Geometry check sheet. Reference: the model listing, model coordinates, mm. A direction names the side the tool comes from. Round coordinates to 2 decimals unless told otherwise and drop trailing zeros. Loops run counter-clockwise (first coordinate to the right, second up) from the corner with the lowest first, then second, coordinate; pieces in that order, holes last. Notation, with made-up numbers: (1, 77.25) - (35, 77.25) arc R16 cw to (35, 83.25) - close; hole circle Ø3 at (33, -10). An arc over 180 degrees is marked (long way). Write item = value, one per line.
Autodesk Inventor part; units mm, degrees
ref_plane "Work Plane1" through (0, 0, -15) normal (0, 0, 1) x (1, 0, 0)
ref_plane "YZ Plane" through (0, 0, 0) normal (1, 0, 0) x (0, 1, 0)
ref_plane "XZ Plane" through (0, 0, 0) normal (0, 1, 0) x (-1, 0, 0)
sketch "Sketch1" plane through (0, 0, 0) normal (0, 0, 1) x (1, 0, 0)
  line L0 (0, 0) -> (25, 0)
  line L1 (25, 0) -> (25, 40)
  line L2 (25, 40) -> (0, 40)
  line L3 (0, 40) -> (0, 0)
  dimension "d1" = 25
  dimension "d2" = 40
  dimension "d3" = 25
extrude "Extrusion1" add sketch "Sketch1" against normal blind 30
sketch "Sketch2" plane through (25, 0, 0) normal (1, 0, 0) x (0, 0, -1)
  line L0 (0, 0) -> (30, 0)
  circle A0 centre (15, 6.56) radius 2.46
extrude "Extrusion2" cut sketch "Sketch2" against normal blind 30
sketch "Sketch3" plane through (0, 0, 0) normal (-1, 0, 0) x (0, 0, 1)
  line L0 (0, 0) -> (-30, 0)
  line L1 (-25.05, 0) -> (-4.95, 0)
  line L2 (-4.95, 0) -> (-4.95, 33.12)
  line L3 (-4.95, 33.12) -> (-25.05, 33.12)
  line L4 (-25.05, 33.12) -> (-25.05, 0)
  dimension "d11" = 20.1
extrude "Extrusion3" cut sketch "Sketch3" against normal blind 20
sketch "Sketch4" plane through (0, 0, 0) normal (0, -1, 0) x (1, 0, 0)
  line L0 (20, -4.95) -> (20, -25.05)
  line L1 (20, -15) -> (25, -15)
  line L2 (25, 0) -> (25, -30)
  line L3 (20, -8.025) -> (25, -8.025)
  line L4 (25, -8.025) -> (25, -21.975)
  line L5 (25, -21.975) -> (20, -21.975)
  line L6 (20, -21.975) -> (20, -8.025)
  line L7 (20, -8.025) -> (25, -21.975) construction
  line L8 (25, -8.025) -> (20, -21.975) construction
  line L9 (25, -12.54) -> (25, -17.46)
  point P0 (0, 0)
  point P1 (22.5, -15)
  dimension "d14" = 13.95
extrude "Extrusion4" add sketch "Sketch4" along normal blind 15
sketch "Sketch5" plane through (20, 0, 0) normal (-1, 0, 0) x (0, 0, 1)
  circle A0 centre (-15, 6.56) radius 2.46
  circle A1 centre (-15, 6.56) radius 4.7025
  circle A2 centre (-15, 6.56) radius 2.46
  circle A3 centre (-15, 6.56) radius 2.46
  point P0 (0, 0)
  dimension "d17" = 9.405
extrude "Extrusion5" cut sketch "Sketch5" against normal blind 2.1
sketch "Sketch6" plane through (25, 0, 0) normal (1, 0, 0) x (0, 0, -1)
  circle A0 centre (15, 6.56) radius 4.7025
  line L0 (15, 6.56) -> (15, 23.56)
  circle A1 centre (15, 23.56) radius 2.46
  point P0 (0, 0)
  dimension "d20" = 17
  dimension "d21" = 4.92
extrude "Extrusion6" cut sketch "Sketch6" against normal blind 10 contours A1
sketch "Sketch7" plane through (20, 0, 0) normal (-1, 0, 0) x (0, 0, 1)
  circle A0 centre (-15, 23.56) radius 2.46
  circle A1 centre (-15, 23.56) radius 4.7025
  point P0 (0, 0)
  dimension "d24" = 9.405
extrude "Extrusion7" cut sketch "Sketch7" against normal blind 2.1
sketch "Sketch9" plane through (25, 0, 0) normal (1, 0, 0) x (0, 0, -1)
  circle A0 centre (15, 6.56) radius 2.46
  circle A1 centre (15, 6.56) radius 2.46
  circle A2 centre (15, 23.56) radius 2.46
  circle A3 centre (15, 23.56) radius 2.46
  line L0 (30, 40) -> (30, 0)
  line L1 (30, 0) -> (30, 40)
  line L2 (30, 40) -> (0, 40)
  line L3 (0, 40) -> (0, 0)
  line L4 (0, 0) -> (8.025, 0)
  line L5 (21.975, 0) -> (21.975, -15)
  line L6 (21.975, -15) -> (8.025, -15)
  line L7 (8.025, -15) -> (8.025, 0)
  line L8 (0, 0) -> (8.025, 0)
  line L9 (21.975, 0) -> (30, 0)
extrude "Extrusion8" add sketch "Sketch9" along normal blind 5
sketch "Sketch10" plane through (0, 40, 0) normal (0, 1, 0) x (1, 0, 0)
  line L0 (0, 30) -> (30, 30)
  line L1 (30, 0) -> (0, 0)
  line L2 (0, 30) -> (30, 30)
  line L3 (30, 30) -> (30, 0)
  line L4 (30, 0) -> (0, 0)
  line L5 (0, 0) -> (0, 30)
extrude "Extrusion9" add sketch "Sketch10" along normal blind 30
sketch "Sketch12" plane through (30, 0, 0) normal (1, 0, 0) x (0, 0, -1)
  circle A0 centre (15, 6.56) radius 2.46
  line L0 (15, 6.56) -> (15, 15.06)
  circle A1 centre (15, 15.06) radius 2.525
  point P0 (0, 0)
  dimension "d31" = 8.5
  dimension "d33" = 5.05
extrude "Extrusion10" cut sketch "Sketch12" against normal blind 30 contours A1
sketch "Sketch14" plane through (0, 0, 0) normal (0, 0, 1) x (1, 0, 0)
  line L0 (30, 70) -> (0, 70)
  line L1 (0, 70) -> (0, 85)
  line L2 (-15, 100) -> (-23, 100)
  line L3 (30, 0) -> (30, 70)
  line L4 (30, 113) -> (30, 70)
  arc A0 (0, 85) -> (-15, 100) centre (-15, 85) ccw
  line L5 (30, 105) -> (30, 100)
  line L6 (-23, 128) -> (15, 128)
  line L7 (-19, 126) -> (-23, 128)
  line L8 (-19, 126) -> (-15, 114)
  line L9 (-19, 102) -> (-23, 100)
  line L10 (-19, 102) -> (-15, 114)
  line L11 (30, 113) -> (15, 128)
  point P0 (0, 0)
  point P1 (0, 100)
  dimension "d47" = 30
  dimension "d54" = 15
  dimension "d69" = 28
extrude "Extrusion12" add sketch "Sketch14" against normal blind 30
sketch "Sketch15" plane through (0, 0, -25.05) normal (-1, 0, 0) x (0, 0, 1)
  line L0 (0, 33.12) -> (20.1, 33.12)
  line L1 (20.1, 33.12) -> (20.1, 0)
  line L2 (0, 33.12) -> (20.1, 33.12)
  line L3 (20.1, 33.12) -> (20.1, 31.1)
  line L4 (20.1, 31.1) -> (0, 31.1)
  line L5 (0, 31.1) -> (0, 33.12)
  point P0 (25.05, 0)
  dimension "d57" = 2.02
extrude "Extrusion13" add sketch "Sketch15" against normal blind 20
sketch "Sketch20" plane through (0, 0, 0) normal (0, 0, 1) x (1, 0, 0)
  arc A0 (0, 85) -> (-15, 100) centre (-15, 85) ccw
  arc A1 (0, 85) -> (-15, 100) centre (-15, 85) ccw
  line L0 (-15, 100) -> (-23, 100)
  line L1 (-15, 100) -> (-23, 100)
  line L2 (-23, 100) -> (-19, 102)
  line L3 (-23, 100) -> (-19, 102)
  line L4 (-19, 102) -> (-15, 114)
  line L5 (-19, 102) -> (-15, 114)
  line L6 (-15, 114) -> (-19, 126)
  line L7 (-15, 114) -> (-19, 126)
  line L8 (-19, 126) -> (-23, 128)
  line L9 (-19, 126) -> (-23, 128)
  line L10 (-23, 128) -> (15, 128)
  line L11 (-23, 128) -> (15, 128)
  line L12 (15, 128) -> (30, 113)
  line L13 (15, 128) -> (30, 113)
  line L14 (30, 113) -> (30, 85)
  line L15 (30, 0) -> (30, 113)
  line L16 (30, 85) -> (0, 85)
  point P0 (0, 0)
extrude "Extrusion14" add sketch "Sketch20" along normal blind 30
ref_plane "Work Plane1" through (0, 0, -15) normal (0, 0, 1) x (1, 0, 0)
mirror "Mirror1" about plane through (0, 0, -15) normal (0, 0, 1) of "Extrusion14"
properties part number "24mm_x_90mm"
(1) Mould release check, pull along Y, two halves, no side actions. Record for faces 5 (the flat face through (10, 15, -4.95)), 6 (the flat face through (10, 31.1, -15)), 7 (the cylindrical face through (25.07, 15.171, -12.477)), 8 (the cylindrical face through (25.995, 7.502, -17.272)): pulls with the +Y half, pulls with the -Y half, needs draft (parallel to the pull), parting line crosses it, or undercut.
Answers follow:
face_5 = needs draft
face_6 = pulls with the -Y half
face_7 = undercut
face_8 = undercut
(2) Set-up check for faces 1 (the flat face through (25, -7, -21.975)), 2 (the cylindrical face through (21.035, 27.525, -12.472)), 3 (the flat face through (-17, 120, -14)), 4 (the flat face through (15, 85, 15)): record each of +Z, -Z, +X, -X, +Y, -Y from which the full face is reachable in a straight line by a thin tool's end or side.
Answers follow:
face_1 = -Z, +X, -X, -Y
face_2 = -X
face_3 = +Z, -Z, -X
face_4 = +Z, +X, -X, -Y
(3) Section check B-B (x = 25.5). Enter the section's corners in (y, z) (3 decimals).
Answers follow:
outline = (-15, -21.975) - (0, -21.975) - (0, -30) - (85, -30) - (85, -60) - (117.5, -60) - (117.5, 30) - (85, 30) - (85, 0) - (0, 0) - (0, -8.025) - (-15, -8.025) - close; hole circle Ø4.92 at (6.56, -15); hole circle Ø5.05 at (15.06, -15); hole circle Ø4.92 at (23.56, -15)
(4) Section check C-C (z = 11). Enter the section's corners in (x, y), then the cut area to 3 significant figures.
Answers follow:
outline = (-23, 100) - (-15, 100) arc R15 cw to (0, 85) - (30, 85) - (30, 113) - (15, 128) - (-23, 128) - (-19, 126) - (-15, 114) - (-19, 102) - close
area = 1,720 mm²
(5) Gauge pin test, flat ends, axial feed: pin 1 (4 mm diameter, centred on x = 14, z = -25, fed in from -Y); pin 2 (6 mm diameter, centred on x = 14.5, y = 21.5, fed in from +Z); pin 3 (7.5 mm diameter, centred on y = 23.56, z = -15, fed in from -X); pin 4 (4.5 mm diameter, centred on y = 6.56, z = -15, fed in from +X). Record the tip position at first contact, or that the pin passes through.
Answers follow:
pin_1 = 0
pin_2 = 0
pin_3 = 22.1
pin_4 = through
(6) Section check D-D (x = 2.5). Enter the section's corners in (y, z).
Answers follow:
outline = (0, -30) - (85, -30) - (85, -60) - (128, -60) - (128, 30) - (85, 30) - (85, 0) - (0, 0) - (0, -4.95) - (31.1, -4.95) - (31.1, -25.05) - (0, -25.05) - close
(7) Section check A-A (y = 15.06). Enter the section's corners in (x, z) (3 decimals).
Answers follow:
outline = (0, -30) - (30, -30) - (30, -17.525) - (20, -17.525) - (20, -25.05) - (0, -25.05) - close; (0, -4.95) - (20, -4.95) - (20, -12.475) - (30, -12.475) - (30, 0) - (0, 0) - close
(8) Scan lines: L1, parallel to Y at x = 27.25, z = -15 (3 decimals); L2, parallel to Y at x = 27.5, z = -15 (3 decimals); L3, parallel to X at y = 51, z = -14. Record each from-to range of solid material in increasing order. Write a range as [from, to].
Answers follow:
L1 = [-15, 4.1], [9.02, 12.535], [17.585, 21.1], [26.02, 115.75]
L2 = [-15, 4.1], [9.02, 12.535], [17.585, 21.1], [26.02, 115.5]
L3 = [0, 30]
